The model under review builds one solid part; all positions refer to its coordinate system, in mm. Face numbers are marked on the shaded views. Round coordinates to 2 decimals unless told otherwise and drop trailing zeros. Loops run counter-clockwise (first coordinate to the right, second up) from the corner with the lowest first, then second, coordinate; pieces in that order, holes last. Notation, with made-up numbers: M -4.75,7.5 L 31.25,7.5 A14 ccw 31.25,21.5 Z; hole C -7.75,59.25 d2. An arc over 180 degrees is marked long. Answer in a Markdown table with one row per item. Add a question column.
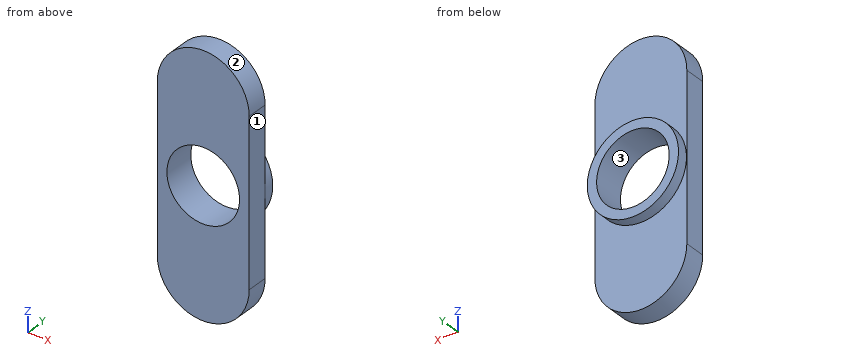
from build123d import *

# Parameters (mm, degrees)
BOSS_EXTRUDE1_DEPTH = 2.54
SKETCH2_R           = 4.2164
CUT_EXTRUDE1_DEPTH  = 2.54
EXTRUDE_THIN1_START = 1.27
SKETCH3_R           = 5.2959
SKETCH3_R_2         = 4.2164
EXTRUDE_THIN1_DEPTH = 1.27


with BuildPart() as part:
    # Sketch1 → Boss-Extrude1 (new body)
    with BuildSketch(Plane(origin=(0, 0, 0), x_dir=(1, 0, 0), z_dir=(0, 1, 0))):
        with BuildLine():
            Line((5.334, 9.525), (5.334, -9.525))
            ThreePointArc((5.334, -9.525), (0, -14.859), (-5.334, -9.525))
            Line((-5.334, -9.525), (-5.334, 9.525))
            ThreePointArc((-5.334, 9.525), (0, 14.859), (5.334, 9.525))
        make_face()
    extrude(amount=BOSS_EXTRUDE1_DEPTH)

    # Sketch2 → Cut-Extrude1 (cut)
    with BuildSketch(Plane(origin=(0, 2.54, 0), x_dir=(1, 0, 0), z_dir=(0, 1, 0))):
        with Locations(Location((0, 0, 0), (0, 0, 270))):
            Circle(SKETCH2_R)
    extrude(amount=-CUT_EXTRUDE1_DEPTH, mode=Mode.SUBTRACT)

    # Sketch3 → Extrude-Thin1 (add)
    with BuildSketch(Plane(origin=(0, 2.54, 0), x_dir=(1, 0, 0), z_dir=(0, 1, 0)).offset(EXTRUDE_THIN1_START)):
        Circle(SKETCH3_R)
        Circle(SKETCH3_R_2, mode=Mode.SUBTRACT)
    extrude(amount=-EXTRUDE_THIN1_DEPTH)


solid = part.part
1. Take a section at A-A, the plane x = -2.5. State the section outline as (y, z) points, and give its area (3 significant figures).
2. Take a section at B-B, the plane y = 3.15. State the section outline as (x, z) points, and give its area (3 significant figures).
3. To check wall thickness, follow probe 1 along X at (y, z) = (2.4, 0); probe 2 along Z at (x, y) = (0, 2.05); probe 3 along X at (y, z) = (1.6, -2). State the ranges of each line that lie inside material, in increasing order.
4. Take a section at C-C, the plane x = 4.75. State the section outline as (y, z) points, and give its area (3 significant figures).
5. For pin 1 Ø2 at (x, z) = (-4, -4.5) entering from -Y; pin 2 Ø1.5 at (y, z) = (3, 11) entering from -X; pin 3 Ø2 at (x, z) = (0, 8) entering from +Y, all flat-tipped, find the tip position at first contact; note any pin that passes through.
6. Take a section at D-D, the plane z = -8.75. State the section outline as (x, y) points, and give its area (3 significant figures).
7. Mouldability with a two-part tool opening along Z and no side actions: class the marked faces 1, 2 and 3 as released by +Z, released by -Z, zero draft, split by the parting line, or undercut.
Check sheet entries:
| question | item | result |
|---|---|---|
| 1 | outline | M 0,-14.24 L 2.54,-14.24 L 2.54,-4.67 L 3.81,-4.67 L 3.81,-3.4 L 0,-3.4 Z; M 0,3.4 L 3.81,3.4 L 3.81,4.67 L 2.54,4.67 L 2.54,14.24 L 0,14.24 Z |
| 1 | area | 58.3 mm^2 |
| 2 | outline | C 0,0 d10.59; hole C 0,0 d8.43 |
| 2 | area | 32.3 mm^2 |
| 3 | probe 1 | x = -5.33 to -4.22, 4.22 to 5.33 |
| 3 | probe 2 | z = -14.86 to -4.22, 4.22 to 14.86 |
| 3 | probe 3 | x = -5.33 to -3.71, 3.71 to 5.33 |
| 4 | outline | M 0,-11.95 L 2.54,-11.95 L 2.54,-2.34 L 3.81,-2.34 L 3.81,2.34 L 2.54,2.34 L 2.54,11.95 L 0,11.95 Z |
| 4 | area | 66.7 mm^2 |
| 5 | pin 1 | stops at y = 0 |
| 5 | pin 2 | stops at x = -5.26 |
| 5 | pin 3 | stops at y = 2.54 |
| 6 | outline | M -5.33,0 L 5.33,0 L 5.33,2.54 L -5.33,2.54 Z |
| 6 | area | 27.1 mm^2 |
| 7 | face 1 | zero draft |
| 7 | face 2 | released by +Z |
| 7 | face 3 | undercut |
